Verification items for the finished model (mm, model axes). Face numbers are marked on the shaded views. Give positions to 0.01 mm unless a question says otherwise; leave off trailing zeros. Write each loop counter-clockwise with the first axis right and the second up, starting at its lowest first coordinate (ties: lowest second). Pieces come first, ordered by that corner, then holes. Notation, with made-up numbers: (-31, 57) - (12, 57) arc R14 ccw to (12, 67) - close; hole circle Ø8 at (-20.5, -18.75). An arc over 180 degrees is marked (long way). Answer as a JSON object with one key per item and string values. Group by question number.
Item 1: Sectioned sample at B-B, the plane x = 0. Record the boundary of the cut face in (y, z), and give its area (3 significant figures).
Item 2: Draft check along Z on the marked faces 1, 2 and 3. Enter one of: +Z half, -Z half, draft (parallel to the pull), parting line (faces both ways), or undercut.
Item 3: Sectioned sample at D-D, the plane x = -3. Record the boundary of the cut face in (y, z), and give its area (3 significant figures).
Item 4: Sectioned sample at C-C, the plane y = 5.25. Record the boundary of the cut face in (x, z).
Item 5: Go/stop test with flat-tipped pins: pin 1 (10 mm diameter, centred on x = -4, z = 3.5, fed in from +Y); pin 2 (8 mm diameter, centred on x = 5, y = 8.5, fed in from +Z); pin 3 (4 mm diameter, centred on x = 7.5, y = 13, fed in from -Z); pin 4 (2 mm diameter, centred on y = 8.5, z = 0.5, fed in from +X). Record where each tip stops, or that it passes through.
Item 6: Scan lines: line 1 along Y through (x, z) = (5.25, 9.5); line 2 along X through (y, z) = (7.25, 0); line 3 along Z through (x, y) = (-2, 18). Record each from-to range of solid material in increasing order. Write a range as [from, to].
Item 7: Sectioned sample at A-A, the plane z = 0. Record the boundary of the cut face in (x, y), and give its area (3 significant figures).
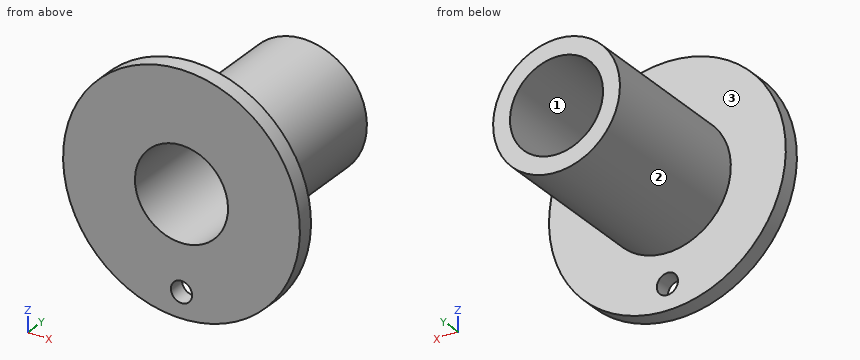
```python
from build123d import *

# Parameters (mm, degrees)
SKETCH1_R           = 14
SKETCH1_R_2         = 5.5
BOSS_EXTRUDE1_DEPTH = 2
SKETCH2_R           = 1.25
CUT_EXTRUDE1_DEPTH  = 2
SKETCH3_R           = 7.5
SKETCH3_R_2         = 5.5
BOSS_EXTRUDE2_DEPTH = 20


with BuildPart() as part:
    # Sketch1 → Boss-Extrude1 (new body)
    with BuildSketch(Plane(origin=(0, 0, 0), x_dir=(1, 0, 0), z_dir=(0, 1, 0))):
        with Locations(Location((0, 0, 0), (0, 0, 270))):
            Circle(SKETCH1_R)
        with Locations(Location((0, 0, 0), (0, 0, 270))):
            Circle(SKETCH1_R_2, mode=Mode.SUBTRACT)
    extrude(amount=BOSS_EXTRUDE1_DEPTH)

    # Sketch2 → Cut-Extrude1 (cut)
    with BuildSketch(Plane(origin=(0, 2, 0), x_dir=(1, 0, 0), z_dir=(0, 1, 0))):
        with Locations(Location((0, 11, 0), (0, 0, 270))):
            Circle(SKETCH2_R)
    extrude(amount=-CUT_EXTRUDE1_DEPTH, mode=Mode.SUBTRACT)

    # Sketch3 → Boss-Extrude2 (add)
    with BuildSketch(Plane(origin=(0, 2, 0), x_dir=(1, 0, 0), z_dir=(0, 1, 0))):
        with Locations(Location((0, 0, 0), (0, 0, 270))):
            Circle(SKETCH3_R)
        with Locations(Location((0, 0, 0), (0, 0, 270))):
            Circle(SKETCH3_R_2, mode=Mode.SUBTRACT)
    extrude(amount=BOSS_EXTRUDE2_DEPTH)


solid = part.part
```
Geometry check:
{
 "1": {"outline": "(0, -14) - (2, -14) - (2, -12.25) - (0, -12.25) - close; (0, -9.75) - (2, -9.75) - (2, -7.5) - (22, -7.5) - (22, -5.5) - (0, -5.5) - close; (0, 5.5) - (22, 5.5) - (22, 7.5) - (2, 7.5) - (2, 14) - (0, 14) - close", "area": "109 mm^2"},
 "2": {"face 1": "undercut", "face 2": "parting line", "face 3": "draft"},
 "3": {"outline": "(0, -13.67) - (2, -13.67) - (2, -6.87) - (22, -6.87) - (22, -4.61) - (0, -4.61) - close; (0, 4.61) - (22, 4.61) - (22, 6.87) - (2, 6.87) - (2, 13.67) - (0, 13.67) - close", "area": "127 mm^2"},
 "4": {"outline": "circle Ø15 at (0, 0); hole circle Ø11 at (0, 0)"},
 "5": {"pin 1": "y = 22", "pin 2": "z = 7.43", "pin 3": "z = -5.1", "pin 4": "x = 7.5"},
 "6": {"line 1": "[0, 2]", "line 2": "[-7.5, -5.5], [5.5, 7.5]", "line 3": "[-7.23, -5.12], [5.12, 7.23]"},
 "7": {"outline": "(-14, 0) - (-5.5, 0) - (-5.5, 22) - (-7.5, 22) - (-7.5, 2) - (-14, 2) - close; (5.5, 0) - (14, 0) - (14, 2) - (7.5, 2) - (7.5, 22) - (5.5, 22) - close", "area": "114 mm^2"}
}
